Print and shaded views of the part. All mm, measured from the part's lowest x, y and z. A direction names the side the tool comes from. Round coordinates to 2 decimals unless told otherwise and drop trailing zeros. Loops run counter-clockwise (first coordinate to the right, second up) from the corner with the lowest first, then second, coordinate; pieces in that order, holes last. Notation, with made-up numbers: (52.5, 30.5) - (94.5, 30.5) arc R14 ccw to (94.5, 55.5) - close; hole circle Ø11 at (69, -37.5). An arc over 180 degrees is marked (long way). Use one line per item in the form item = value.
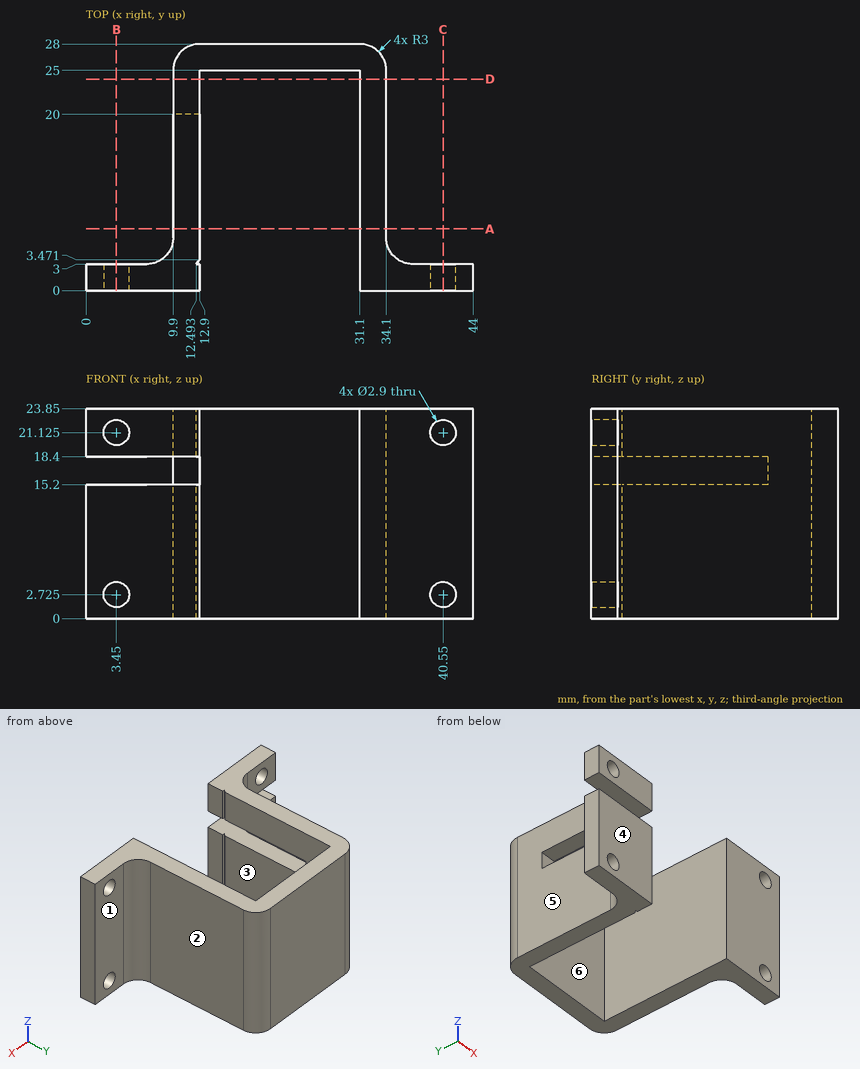
1. Wall check: probe 1 along X at (y, z) = (24.25, 2.5); probe 2 along Y at (x, z) = (16, 8); probe 3 along X at (y, z) = (6.5, 18). Give the ranges that are in metal, low to high.
Geometry check:
probe_1 = 9.9 to 12.9, 31.1 to 34.1
probe_2 = 25 to 28
probe_3 = 31.1 to 34.1
2. Flat gauge pins, fed straight in: pin 1 (4 mm diameter, centred on x = 28, y = 9.5, fed in from -Z); pin 2 (5.5 mm diameter, centred on y = 13, z = 12, fed in from -X); pin 3 (1 mm diameter, centred on y = 12, z = 13.5, fed in from +X); pin 4 (6 mm diameter, centred on x = 4.5, z = 21.5, fed in from +Y). Where does each tip first touch, or does it go through?
Geometry check:
pin_1 = through
pin_2 = 9.9
pin_3 = 34.1
pin_4 = 3.06
3. Cut at B-B, the plane x = 3.45. Give the cut face in (y, z) (3 decimals).
Geometry check:
outline = (0, 0) - (3, 0) - (3, 1.275) - (0, 1.275) - close; (0, 4.175) - (3, 4.175) - (3, 15.2) - (0, 15.2) - close; (0, 18.4) - (3, 18.4) - (3, 19.675) - (0, 19.675) - close; (0, 22.575) - (3, 22.575) - (3, 23.85) - (0, 23.85) - close
4. Cut at D-D, the plane y = 24. Give the cut face in (x, z).
Geometry check:
outline = (9.9, 0) - (12.9, 0) - (12.9, 23.85) - (9.9, 23.85) - close; (31.1, 0) - (34.1, 0) - (34.1, 23.85) - (31.1, 23.85) - close
5. Cut at C-C, the plane x = 40.55. Give the cut face in (y, z) (3 decimals).
Geometry check:
outline = (0, 0) - (3, 0) - (3, 1.275) - (0, 1.275) - close; (0, 4.175) - (3, 4.175) - (3, 19.675) - (0, 19.675) - close; (0, 22.575) - (3, 22.575) - (3, 23.85) - (0, 23.85) - close
6. Pull direction X, two halves, no side cores. Call the marked faces 1, 2 and 3: +X half, -X half, draft (parallel to the pull), parting line (faces both ways), or undercut.
Geometry check:
face_1 = draft
face_2 = +X half
face_3 = undercut
7. Tool access for the marked faces 4, 5 and 6: list every direction of +Z, -Z, +X, -X, +Y, -Y with a clear straight run to the whole face (end or side of a thin tool).
Geometry check:
face_4 = +Z, -Z, +X, -X, -Y
face_5 = +Z, -Z, -X, +Y
face_6 = +Z, -Z, -Y
8. Cut at A-A, the plane y = 7. Give the cut face in (x, z), plus the area to 4 significant figures.
Geometry check:
outline = (9.9, 0) - (12.9, 0) - (12.9, 15.2) - (9.9, 15.2) - close; (9.9, 18.4) - (12.9, 18.4) - (12.9, 23.85) - (9.9, 23.85) - close; (31.1, 0) - (34.1, 0) - (34.1, 23.85) - (31.1, 23.85) - close
area = 133.5 mm^2
